For this review, take the finished solid that the model builds, in its own axes (mm). A direction names the side the tool comes from. Give positions to 0.01 mm unless a question says otherwise; leave off trailing zeros. Write each loop counter-clockwise with the first axis right and the second up, starting at its lowest first coordinate (ties: lowest second). Pieces come first, ordered by that corner, then holes. Notation, with made-up numbers: M 53,18 L 88,18 A11 cw 88,38 Z; hole C 57,-28 d5. An arc over 180 degrees is marked long. Use one line per item in the form item = value. Start each with the question number.
Q1. Mouldability with a two-part tool opening along Z and no side actions: class faces 3 (the flat face through (3, 100, -59.69)), 4 (the flat face through (0, 61, -23)), 5 (the cylindrical face through (3.219, 78.346, -17.98)) as released by +Z, released by -Z, zero draft, split by the parting line, or undercut.
Q2. Tool access review of faces 1 (the flat face through (3, 80.01, -50)), 2 (the flat face through (3, 120.65, -30)): name each direction out of +Z, -Z, +X, -X, +Y, -Y from which nothing blocks a thin tool from reaching the whole face with its end or side.
Q3. Clearance check with flat-ended pins moving along their axes: pin 1 Ø3 at (x, y) = (3, 39) entering from -Z; pin 2 Ø4 at (y, z) = (52.39, -20.32) entering from +X. State where each tip first meets the part, or that it passes through.
Q4. For probe 1 along Y at (x, z) = (3.75, -20); probe 2 along Y at (x, z) = (2.5, -17.5); probe 3 along Y at (x, z) = (4.25, -53), list the stretches that pass through material, from the lowest coordinate up. Write a range as [from, to].
Q5. Consider section B-B on y = 76.2. Write out the cut boundary in (x, z) (3 decimals).
Q6. Consider section A-A on y = 95.25. Give the number of separate pieces and of enclosed holes in the cut face, and give its area (3 significant figures).
```python
from build123d import *

# Parameters (mm, degrees)
BOSS_EXTRUDE1_DEPTH = 6.35
SKETCH3_R           = 3.175
CUT_EXTRUDE1_DEPTH  = 6.35


with BuildPart() as part:
    # Sketch1 → Boss-Extrude1 (new body)
    with BuildSketch(Plane(origin=(0, 0, 0), x_dir=(0, 0, -1), z_dir=(1, 0, 0))):
        Polygon((0, 0), (40.64, 0), (40.64, 80.01), (59.69, 80.01), (59.69, 120.65), (40.64, 120.65), (0, 120.65), align=None)
    extrude(amount=BOSS_EXTRUDE1_DEPTH)

    # Sketch3 → Cut-Extrude1 (cut)
    with BuildSketch(Plane(origin=(6.35, 0, 0), x_dir=(0, 0, -1), z_dir=(1, 0, 0))):
        with Locations((20.32, 19.05)):
            Circle(SKETCH3_R)
        with Locations((20.32, 52.3875)):
            Circle(SKETCH3_R)
        with Locations((20.32, 76.2)):
            Circle(SKETCH3_R)
        with Locations((20.32, 95.25)):
            Circle(SKETCH3_R)
        with Locations((44.1325, 95.25)):
            Circle(SKETCH3_R)
    extrude(amount=-CUT_EXTRUDE1_DEPTH, mode=Mode.SUBTRACT)


solid = part.part
```
Working result:
q1.face_3 = released by -Z
q1.face_4 = zero draft
q1.face_5 = undercut
q2.face_1 = -Z, +X, -X, -Y
q2.face_2 = +Z, -Z, +X, -X, +Y
q3.pin_1 = -40.64
q3.pin_2 = through
q4.probe_1 = [0, 15.89], [22.21, 49.23], [55.55, 73.04], [79.36, 92.09], [98.41, 120.65]
q4.probe_2 = [0, 17.59], [20.51, 50.93], [53.85, 74.74], [77.66, 93.79], [96.71, 120.65]
q4.probe_3 = [80.01, 120.65]
q5.outline = M 0,-40.64 L 6.35,-40.64 L 6.35,-23.495 L 0,-23.495 Z; M 0,-17.145 L 6.35,-17.145 L 6.35,0 L 0,0 Z
q6.separate_pieces = 3
q6.enclosed_holes = 0
q6.area = 298 mm²
